```python
from build123d import *

# Parameters (mm, degrees)
F0_W     = 939.8
F0_H     = 977.9
F1_DEPTH = 6.35
F2_W     = 762
F2_H     = 450.85
F2_W_2   = 609.6
F2_H_2   = 266.7
F3_DEPTH = 12.701


with BuildPart() as f1:
    # F0 (on Right) → F1 (new body, symmetric)
    with BuildSketch(Plane.YZ):
        Rectangle(F0_W, F0_H)
    extrude(amount=F1_DEPTH, both=True)

    # F2 (on face) → F3 (cut, through all)
    with BuildSketch(Plane.YZ.offset(6.35)):
        with Locations((0, -155.575)):
            Rectangle(F2_W, F2_H)
        with Locations((0, 317.5)):
            Rectangle(F2_W_2, F2_H_2)
    extrude(amount=-F3_DEPTH, mode=Mode.SUBTRACT)


solid = f1.part
```
The model under review builds one solid part; all positions refer to its coordinate system, in mm. Give positions to 0.01 mm unless a question says otherwise; leave off trailing zeros. Write each loop counter-clockwise with the first axis right and the second up, starting at its lowest first coordinate (ties: lowest second). Pieces come first, ordered by that corner, then holes. Notation, with made-up numbers: M 3,62.5 L 31,62.5 A12 ccw 31,80.5 Z; hole C 47,28 d6. An arc over 180 degrees is marked long. Answer in a Markdown table with one row per item.
Item 1: Add section C-C on y = 317. Give the boundary of the cut face in (x, z), plus the area to 3 significant figures.
Check sheet entries:
| item | result |
|---|---|
| outline | M -6.35,-488.95 L 6.35,-488.95 L 6.35,-381 L -6.35,-381 Z; M -6.35,69.85 L 6.35,69.85 L 6.35,488.95 L -6.35,488.95 Z |
| area | 6,690 mm2 |
Item 2: Add section D-D on x = 4.25. Give the boundary of the cut face in (y, z).
Check sheet entries:
| item | result |
|---|---|
| outline | M -469.9,-488.95 L 469.9,-488.95 L 469.9,488.95 L -469.9,488.95 Z; hole M -381,-381 L 381,-381 L 381,69.85 L -381,69.85 Z; hole M -304.8,184.15 L 304.8,184.15 L 304.8,450.85 L -304.8,450.85 Z |
Item 3: For line 1 along Z through (x, y) = (5.5, 103.5); line 2 along Y through (x, z) = (5.75, -160); line 3 along Y through (x, z) = (1, 338), list the stretches that pass through material, from the lowest coordinate up.
Check sheet entries:
| item | result |
|---|---|
| line 1 | -488.95 to -381, 69.85 to 184.15, 450.85 to 488.95 |
| line 2 | -469.9 to -381, 381 to 469.9 |
| line 3 | -469.9 to -304.8, 304.8 to 469.9 |
Item 4: Add section A-A on y = -11.5. Give the boundary of the cut face in (x, z), plus the area to 3 significant figures.
Check sheet entries:
| item | result |
|---|---|
| outline | M -6.35,-488.95 L 6.35,-488.95 L 6.35,-381 L -6.35,-381 Z; M -6.35,69.85 L 6.35,69.85 L 6.35,184.15 L -6.35,184.15 Z; M -6.35,450.85 L 6.35,450.85 L 6.35,488.95 L -6.35,488.95 Z |
| area | 3,310 mm2 |
Item 5: Add section B-B on z = -75.5. Give the boundary of the cut face in (x, y), plus the area to 3 significant figures.
Check sheet entries:
| item | result |
|---|---|
| outline | M -6.35,-469.9 L 6.35,-469.9 L 6.35,-381 L -6.35,-381 Z; M -6.35,381 L 6.35,381 L 6.35,469.9 L -6.35,469.9 Z |
| area | 2,260 mm2 |
